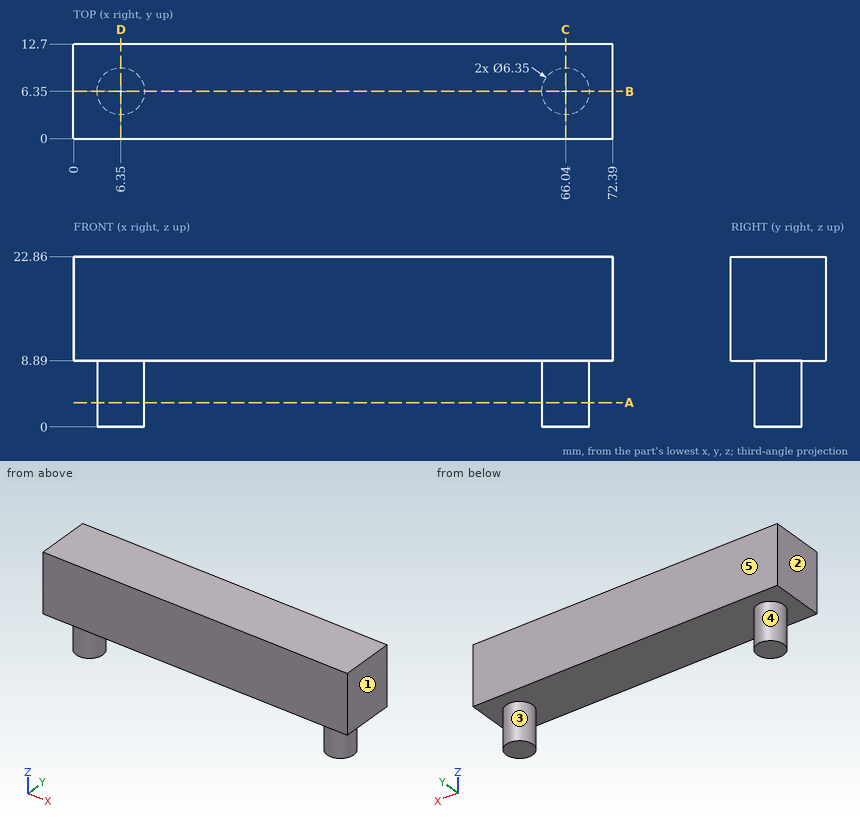
Verification items for this drawing (mm, ordinates from the low corner). A direction names the side the tool comes from. Give positions to 0.01 mm unless a question says otherwise; leave off trailing zeros. Loops run counter-clockwise (first coordinate to the right, second up) from the corner with the lowest first, then second, coordinate; pieces in that order, holes last. Notation, with made-up numbers: M 10,-39 L 25,-39 A5 cw 25,-34 Z; hole C 31.5,81.5 d11. An arc over 180 degrees is marked long. Answer as CSV lines item,"result".
Item 1: Cross-section at B-B on y = 6.35. Record the cut outline in (x, z) (3 decimals).
Values:
outline,"M 0,8.89 L 3.175,8.89 L 3.175,0 L 9.525,0 L 9.525,8.89 L 62.865,8.89 L 62.865,0 L 69.215,0 L 69.215,8.89 L 72.39,8.89 L 72.39,22.86 L 0,22.86 Z"
Item 2: Cross-section at A-A on z = 3.25. Record the cut outline in (x, y) (3 decimals), and give its area (3 significant figures).
Values:
outline,"C 6.35,6.35 d6.35; C 66.04,6.35 d6.35"
area,"63.3 mm²"
Item 3: Depth check by flat-ended pin: P1, Ø8, axis at x = 8.5, z = 12.5, coming from the -Y side; P2, Ø4, axis at x = 32.5, y = 9.5, coming from the -Z side; P3, Ø2, axis at y = 2, z = 7.5, coming from the -X side. Enter the tip coordinate at first touch or a pass-through.
Values:
P1,"stops at y = 0"
P2,"stops at z = 8.89"
P3,"passes through"
Item 4: Material ranges on line 1 (X direction, y = 6.25, z = 4.75); line 2 (Z direction, x = 3, y = 3.5); line 3 (X direction, y = 7.75, z = 2), recorded low to high.
Values:
line 1,"x = 3.18 to 9.52, 62.87 to 69.21"
line 2,"z = 8.89 to 22.86"
line 3,"x = 3.5 to 9.2, 63.19 to 68.89"
Item 5: Release check for a two-part mould opening along X. For the marked faces 1, 2 and 3 record: pulls with the +X half, pulls with the -X half, needs draft (parallel to the pull), parting line crosses it, or undercut.
Values:
face 1,"pulls with the +X half"
face 2,"pulls with the -X half"
face 3,"undercut"
Item 6: Access from +Z, -Z, +X, -X, +Y, -Y to the whole of each face (thin tool, end or side, straight path). Record for the marked faces 4 and 5.
Values:
face 4,"-Z"
face 5,"+Z, -Z, +X, -X, +Y"
Item 7: Cross-section at C-C on x = 66.04. Record the cut outline in (y, z) (3 decimals).
Values:
outline,"M 0,8.89 L 3.175,8.89 L 3.175,0 L 9.525,0 L 9.525,8.89 L 12.7,8.89 L 12.7,22.86 L 0,22.86 Z"
